For this review, take the finished solid that the model builds, in its own axes (mm). A direction names the side the tool comes from. Give positions to 0.01 mm unless a question says otherwise; leave off trailing zeros. Loops run counter-clockwise (first coordinate to the right, second up) from the corner with the lowest first, then second, coordinate; pieces in that order, holes last. Notation, with made-up numbers: (22, 17) - (64, 17) arc R22 cw to (64, 32) - close; hole circle Ø6 at (17, 24). An arc over 180 degrees is marked (long way). Answer as CSV lines item,"result".
from build123d import *

# Parameters (mm, degrees)
SKETCH_W      = 112
SKETCH_H      = 73.4
SKETCH_W_2    = 107
SKETCH_H_2    = 68.4
PAD_DEPTH     = 15
SKETCH001_W   = 6.5
SKETCH001_H   = 6.5
SKETCH001_W_2 = 7.5
PAD001_DEPTH  = 2
SKETCH002_R   = 1.5
POCKET_DEPTH  = 2
SKETCH003_W   = 2
SKETCH003_H   = 73.4
PAD002_DEPTH  = 2


with BuildPart() as part:
    # Sketch → Pad (new body)
    with BuildSketch(Plane.XY):
        Rectangle(SKETCH_W, SKETCH_H)
        Rectangle(SKETCH_W_2, SKETCH_H_2, mode=Mode.SUBTRACT)
    extrude(amount=PAD_DEPTH)

    # Sketch001 (on Face9 of Pad) → Pad001 (join)
    with BuildSketch(Plane(origin=(0, 0, 0), x_dir=(1, 0, 0), z_dir=(0, 0, -1))):
        with Locations((-50.25, 30.95)):
            Rectangle(SKETCH001_W, SKETCH001_H)
        with Locations((-49.75, -30.95)):
            Rectangle(SKETCH001_W_2, SKETCH001_H)
        with Locations((50.25, 30.95)):
            Rectangle(SKETCH001_W, SKETCH001_H)
        with Locations((50.25, -30.95)):
            Rectangle(SKETCH001_W, SKETCH001_H)
    extrude(amount=-PAD001_DEPTH)

    # Sketch002 (on Face22 of Pad001) → Pocket (cut)
    with BuildSketch(Plane(origin=(0, 0, 0), x_dir=(1, 0, 0), z_dir=(0, 0, -1))):
        with Locations((-50.25, 30.75)):
            Circle(SKETCH002_R)
        with Locations((50.25, -30.75)):
            Circle(SKETCH002_R)
        with Locations((-49.75, -30.75)):
            Circle(SKETCH002_R)
        with Locations((50.25, 30.75)):
            Circle(SKETCH002_R)
    extrude(amount=-POCKET_DEPTH, mode=Mode.SUBTRACT)

    # Sketch003 (on Face9 of Pad) → Pad002 (join)
    with BuildSketch(Plane(origin=(0, 0, 0), x_dir=(1, 0, 0), z_dir=(0, 0, -1))):
        with Locations((-20.205, 0)):
            Rectangle(SKETCH003_W, SKETCH003_H)
        with Locations((20.205, 0)):
            Rectangle(SKETCH003_W, SKETCH003_H)
    extrude(amount=PAD002_DEPTH)


solid = part.part
1) Consider section D-D on z = 6.75. Write out the cut boundary in (x, y).
From the geometry:
outline,"(-56, -36.7) - (56, -36.7) - (56, 36.7) - (-56, 36.7) - close; hole (-53.5, -34.2) - (53.5, -34.2) - (53.5, 34.2) - (-53.5, 34.2) - close"
2) Consider section C-C on y = 11.5. Write out the cut boundary in (x, z) (3 decimals).
From the geometry:
outline,"(-56, 0) - (-53.5, 0) - (-53.5, 15) - (-56, 15) - close; (-21.205, -2) - (-19.205, -2) - (-19.205, 0) - (-21.205, 0) - close; (19.205, -2) - (21.205, -2) - (21.205, 0) - (19.205, 0) - close; (53.5, 0) - (56, 0) - (56, 15) - (53.5, 15) - close"
3) Insertion check: P1, Ø1, axis at x = 20, y = 6, coming from the +Z side; P2, Ø12, axis at x = -10.5, y = -0.5, coming from the +Z side; P3, Ø3.5, axis at x = 50.25, y = -30.75, coming from the +Z side; P4, Ø2, axis at x = 8, y = -35.5, coming from the -Z side. Each pin has a flat end and moves straight along its axis. Give the tip position at first contact, or say it passes through.
From the geometry:
P1,"stops at z = 0"
P2,"passes through"
P3,"stops at z = 2"
P4,"stops at z = 0"
4) Draft analysis for pull direction X (two halves, no side actions). For faces 4 (the flat face through (56, -1, 7)), 5 (the flat face through (50.2, -32.4, 2)), 6 (the flat face through (54, 3, 0)), state which applies: pulls with the +X half, pulls with the -X half, needs draft (parallel to the pull), parting line crosses it, or undercut.
From the geometry:
face 4,"pulls with the +X half"
face 5,"undercut"
face 6,"needs draft"
5) Consider section A-A on x = 50.25. Write out the cut boundary in (y, z), and give its area (3 significant figures).
From the geometry:
outline,"(-36.7, 0) - (-32.25, 0) - (-32.25, 2) - (-34.2, 2) - (-34.2, 15) - (-36.7, 15) - close; (-29.25, 0) - (-27.7, 0) - (-27.7, 2) - (-29.25, 2) - close; (27.7, 0) - (29.25, 0) - (29.25, 2) - (27.7, 2) - close; (32.25, 0) - (36.7, 0) - (36.7, 15) - (34.2, 15) - (34.2, 2) - (32.25, 2) - close"
area,"89.0 mm^2"
6) Machinability: for faces 1 (the cylindrical face through (48.75, -30.82, 0.99)), 2 (the flat face through (0, 35, 0)), 3 (the flat face through (-50.3, -32.4, 2)), which of the approach directions +Z, -Z, +X, -X, +Y, -Y give a long, thin tool a straight path to every point of the face, cutting with its end or side? Answer none if there is none.
From the geometry:
face 1,"+Z, -Z"
face 2,"-Z, +Y, -Y"
face 3,"+Z"
7) Consider section B-B on y = 30.75. Write out the cut boundary in (x, z) (3 decimals), and give its area (3 significant figures).
From the geometry:
outline,"(-56, 0) - (-51.25, 0) - (-51.25, 2) - (-53.5, 2) - (-53.5, 15) - (-56, 15) - close; (-48.25, 0) - (-46, 0) - (-46, 2) - (-48.25, 2) - close; (-21.205, -2) - (-19.205, -2) - (-19.205, 0) - (-21.205, 0) - close; (19.205, -2) - (21.205, -2) - (21.205, 0) - (19.205, 0) - close; (47, 0) - (48.75, 0) - (48.75, 2) - (47, 2) - close; (51.75, 0) - (56, 0) - (56, 15) - (53.5, 15) - (53.5, 2) - (51.75, 2) - close"
area,"99.0 mm^2"
8) Wall thickness on line 1 (X direction, y = 30.75, z = 1.4); line 2 (X direction, y = -30.75, z = 1.55); line 3 (Y direction, x = 50.25, z = 0.7): over which ranges is each line inside the solid? List them lowest first. Write a range as from..to.
From the geometry:
line 1,"x = -56..-51.25, -48.25..-46, 47..48.75, 51.75..56"
line 2,"x = -56..-51.75, -48.75..-47, 47..48.75, 51.75..56"
line 3,"y = -36.7..-32.25, -29.25..-27.7, 27.7..29.25, 32.25..36.7"
